CAD build for the part. Positions are in the model's coordinates, mm. Face numbers are marked on the shaded views. A direction names the side the tool comes from. Give positions to 0.01 mm unless a question says otherwise; leave off trailing zeros. Write each loop counter-clockwise with the first axis right and the second up, starting at its lowest first coordinate (ties: lowest second). Pieces come first, ordered by that corner, then holes. Notation, with made-up numbers: M 67.25,45.5 L 115.25,45.5 A17 ccw 115.25,75.5 Z; hole C 65.25,48.5 d3. An arc over 180 degrees is marked long. One line per question, with ' | ' between items. Start each with the question number.
1. Cut at B-B, the plane z = -1.5. Write the cut outline in (x, y), then the cut area to 3 significant figures.
2. Flat gauge pins, fed straight in: pin 1 (1 mm diameter, centred on x = 4.5, z = -1.5, fed in from -Y); pin 2 (3 mm diameter, centred on x = 5, z = -3.5, fed in from -Y); pin 3 (1.5 mm diameter, centred on y = 3.5, z = -4, fed in from +X). Where does each tip first touch, or does it go through?
3. Wall check: L1, parallel to Y at x = 0, z = -1.7; L2, parallel to Y at x = 1.25, z = -0.35; L3, parallel to X at y = -1, z = -1.45. Give the ranges that are in metal, low to high.
4. Pull direction Y, two halves, no side cores. Call the marked faces 1, 2, 3 and 4: released by +Y, released by -Y, zero draft, split by the parting line, or undercut.
5. Cut at D-D, the plane x = -5. Write the cut outline in (y, z).
6. Which spindle directions (+Z, -Z, +X, -X, +Y, -Y) get a long thin tool onto all of the face, cutting with end or side? Do the marked faces 5 and 6. Say none if no direction does.
7. Cut at C-C, the plane y = 3. Write the cut outline in (x, z), then the cut area to 3 significant figures.
8. Cut at A-A, the plane x = 0. Write the cut outline in (y, z).
```python
from build123d import *

# Parameters (mm, degrees)
F0_R     = 6.1976
F1_DEPTH = 5.842
F3_DEPTH = 5.842


# Not quite as in the source:
# - a feature names something its author has since deleted; it is built from what else it names


with BuildPart() as f1:
    # F0 (on Top) → F1 (new body)
    with BuildSketch(Plane.XY):
        with BuildLine():
            ThreePointArc((-12.7, 0), (0, -12.7), (12.7, 0))
            ThreePointArc((12.7, 0), (0, 12.7), (-12.7, 0))
        make_face()
        Circle(F0_R, mode=Mode.SUBTRACT)
        with BuildLine():
            Line((12.7, -12.7), (12.7, 0))
            ThreePointArc((12.7, 0), (0, -12.7), (-12.7, 0))
            Line((-12.7, 0), (-12.7, -12.7))
            ThreePointArc((-12.7, -12.7), (0, -25.4), (12.7, -12.7))
        make_face()
    extrude(amount=-F1_DEPTH)

    # F2 (on face) → F3 (cut, through all)
    with BuildSketch(Plane.XY):
        with BuildLine():
            Line((12.7, -9.3726), (-2.921, -9.3726))
            Line((-2.921, -9.3726), (-2.921, -15.7226))
            Line((-2.921, -15.7226), (2.921, -15.7226))
            Line((2.921, -15.7226), (2.921, -15.4051))
            Line((2.921, -15.4051), (12.3350674599, -15.7226))
            ThreePointArc((12.3350674599, -15.7226), (12.6084367933, -14.2222751491), (12.7, -12.7))
            Line((12.7, -12.7), (12.7, -9.3726))
        make_face()
    extrude(amount=-F3_DEPTH, mode=Mode.SUBTRACT)


solid = f1.part
```
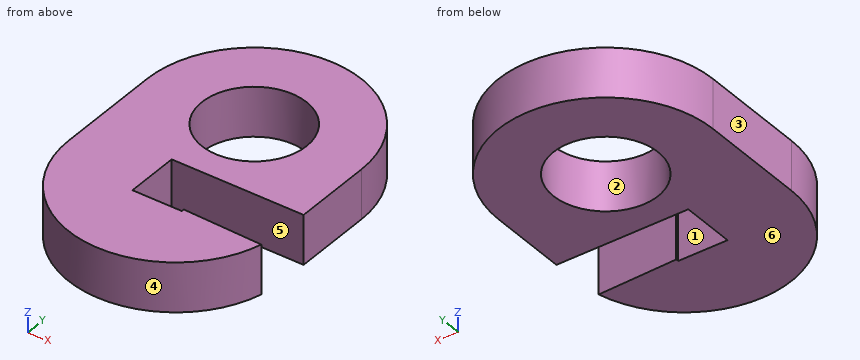
Here are the results:
1) outline: M -12.7,-12.7 A12.7 ccw 12.34,-15.72 L 2.92,-15.41 L 2.92,-15.72 L -2.92,-15.72 L -2.92,-9.37 L 12.7,-9.37 L 12.7,0 A12.7 ccw -12.7,0 Z; hole C 0,0 d12.4 | area: 611 mm^2
2) pin 1: y = -24.75 | pin 2: y = -24.91 | pin 3: x = 12.4
3) L1: -25.4 to -15.72, -9.37 to -6.2, 6.2 to 12.7 | L2: -25.34 to -15.72, -9.37 to -6.07, 6.07 to 12.64 | L3: -12.7 to -6.12, 6.12 to 12.7
4) face 1: undercut | face 2: undercut | face 3: zero draft | face 4: released by -Y
5) outline: M -24.37,-5.84 L -3.66,-5.84 L -3.66,0 L -24.37,0 Z; M 3.66,-5.84 L 11.67,-5.84 L 11.67,0 L 3.66,0 Z
6) face 5: +Z, -Z, +X | face 6: -Z, +X, -X, +Y, -Y
7) outline: M -12.34,-5.84 L -5.42,-5.84 L -5.42,0 L -12.34,0 Z; M 5.42,-5.84 L 12.34,-5.84 L 12.34,0 L 5.42,0 Z | area: 80.8 mm^2
8) outline: M -25.4,-5.84 L -15.72,-5.84 L -15.72,0 L -25.4,0 Z; M -9.37,-5.84 L -6.2,-5.84 L -6.2,0 L -9.37,0 Z; M 6.2,-5.84 L 12.7,-5.84 L 12.7,0 L 6.2,0 Z
